from build123d import *

# Parameters (mm, degrees)
BOSS_EXTRUDE1_DEPTH = 6
SKETCH2_R           = 7.5
BOSS_EXTRUDE2_DEPTH = 24
BOSS_EXTRUDE3_DEPTH = 6
SKETCH4_R           = 6.75
CUT_EXTRUDE1_DEPTH  = 44.338781709
SKETCH5_R           = 2.25
CUT_EXTRUDE2_DEPTH  = 13
CHAMFER1_SIZE       = 1
CHAMFER2_SIZE       = 2
SKETCH6_R           = 2
CUT_EXTRUDE3_DEPTH  = 44.338781709


with BuildPart() as part:
    # Sketch1 → Boss-Extrude1 (new body)
    with BuildSketch(Plane.XY):
        with BuildLine():
            Line((-13.5, 0), (-13.5, -20))
            Line((-13.5, -20), (13.5, -20))
            Line((13.5, -20), (13.5, 0))
            ThreePointArc((13.5, 0), (0, 13.5), (-13.5, 0))
        make_face()
    extrude(amount=BOSS_EXTRUDE1_DEPTH)

    # Sketch2 → Boss-Extrude2 (add)
    with BuildSketch(Plane.XY.offset(6)):
        Circle(SKETCH2_R)
    extrude(amount=BOSS_EXTRUDE2_DEPTH)

    # Sketch3 → Boss-Extrude3 (add)
    with BuildSketch(Plane.XY.offset(30)):
        with BuildLine():
            Line((-13.5, 0), (-13.5, -20))
            Line((-13.5, -20), (13.5, -20))
            Line((13.5, -20), (13.5, 0))
            ThreePointArc((13.5, 0), (0, 13.5), (-13.5, 0))
        make_face()
    extrude(amount=BOSS_EXTRUDE3_DEPTH)

    # Sketch4 → Cut-Extrude1 (cut, through all)
    with BuildSketch(Plane.XY.offset(36)):
        Circle(SKETCH4_R)
    extrude(amount=-CUT_EXTRUDE1_DEPTH, mode=Mode.SUBTRACT)

    # Sketch5 → Cut-Extrude2 (cut)
    with BuildSketch(Plane.XZ.offset(20)):
        with Locations((-5, 33)):
            Circle(SKETCH5_R)
        with Locations((5, 33)):
            Circle(SKETCH5_R)
        with Locations((-5, 3)):
            Circle(SKETCH5_R)
        with Locations((5, 3)):
            Circle(SKETCH5_R)
    extrude(amount=-CUT_EXTRUDE2_DEPTH, mode=Mode.SUBTRACT)

    # Chamfer1
    # the kernel refuses this chamfer: 1 mm, written as the material it takes off along each edge
    with BuildSketch(Plane(origin=(5, -20, 33), x_dir=(1, 0, 0), z_dir=(0, 0, -1))) as chamfer1_piece_1:
        Polygon((2.25 + CHAMFER1_SIZE, 0), (2.25, -CHAMFER1_SIZE), (2.25, 0), align=None)
    revolve(axis=Axis((5, -20, 33), (0, -1, 0)), mode=Mode.SUBTRACT)
    with BuildSketch(Plane(origin=(-5, -20, 3), x_dir=(1, 0, 0), z_dir=(0, 0, -1))) as chamfer1_piece_2:
        Polygon((2.25 + CHAMFER1_SIZE, 0), (2.25, -CHAMFER1_SIZE), (2.25, 0), align=None)
    revolve(axis=Axis((-5, -20, 3), (0, -1, 0)), mode=Mode.SUBTRACT)
    with BuildSketch(Plane(origin=(5, -20, 3), x_dir=(1, 0, 0), z_dir=(0, 0, -1))) as chamfer1_piece_3:
        Polygon((2.25 + CHAMFER1_SIZE, 0), (2.25, -CHAMFER1_SIZE), (2.25, 0), align=None)
    revolve(axis=Axis((5, -20, 3), (0, -1, 0)), mode=Mode.SUBTRACT)
    with BuildSketch(Plane(origin=(-5, -20, 33), x_dir=(1, 0, 0), z_dir=(0, 0, -1))) as chamfer1_piece_4:
        Polygon((2.25 + CHAMFER1_SIZE, 0), (2.25, -CHAMFER1_SIZE), (2.25, 0), align=None)
    revolve(axis=Axis((-5, -20, 33), (0, -1, 0)), mode=Mode.SUBTRACT)

    # Chamfer2
    chamfer2_edges = [part.edges().sort_by_distance(p)[0] for p in [
        (13.5, -10, 6),
        (0, 13.5, 30),
        (-13.5, -10, 30),
        (13.5, -10, 30),
        (0, 13.5, 36),
        (-13.5, -10, 36),
        (13.5, -10, 36),
        (0, 13.5, 6),
        (13.5, -10, 0),
        (-13.5, -10, 0),
        (0, 13.5, 0),
        (-13.5, -10, 6),
    ]]
    chamfer(chamfer2_edges, length=CHAMFER2_SIZE)

    # Sketch6 → Cut-Extrude3 (cut, through all)
    with BuildSketch(Plane.XY.offset(36)):
        with Locations(Location((-10, 0, 0), (0, 0, 221.409622109))):
            Circle(SKETCH6_R)
    extrude(amount=-CUT_EXTRUDE3_DEPTH, mode=Mode.SUBTRACT)


solid = part.part
The model under review builds one solid part; all positions refer to its coordinate system, in mm. A direction names the side the tool comes from. Round coordinates to 2 decimals unless told otherwise and drop trailing zeros. Write each loop counter-clockwise with the first axis right and the second up, starting at its lowest first coordinate (ties: lowest second). Pieces come first, ordered by that corner, then holes. Notation, with made-up numbers: M 59.25,38 L 101.25,38 A23 cw 101.25,59 Z; hole C 9,37 d7. An arc over 180 degrees is marked long. Use a Markdown table: item, result. Add a question column.
Q1. Insertion check: pin 1 (2.5 mm diameter, centred on x = -5, z = 33, fed in from -Y); pin 2 (7 mm diameter, centred on x = 5, z = 3, fed in from -Y); pin 3 (2 mm diameter, centred on x = -4, z = 4, fed in from -Y); pin 4 (10 mm diameter, centred on y = -4, z = 11.5, fed in from +X). Each pin has a flat end and moves straight along its axis. Give the tip position at first contact, or say it passes through.
Q2. To check wall thickness, follow line 1 (Z direction, x = -5, y = -10.75); line 2 (X direction, y = -18.5, z = 2.5); line 3 (Y direction, x = 0, z = 15.5). State the ranges of each line that lie inside material, in increasing order.
Q3. We need section B-B, the plane z = 33. State the section outline as (x, y) points.
Q4. We need section A-A, the plane y = -16.5. State the section outline as (x, z) points, plus the area to 3 significant figures.
Q5. We need section C-C, the plane y = -3. State the section outline as (x, z) points, plus the area to 3 significant figures.
Q6. The part is to be moulded in two halves that separate along Z. For faces 4 (the face through (0, -8, 0)), 5 (the face through (-13.5, -10, 3)), 6 (the face through (5, -7, 3)), say which applies: pulls with the +Z half, pulls with the -Z half, needs draft (parallel to the pull), parting line crosses it, or undercut.
Q7. Machinability: for faces 1 (the face through (0, -8, 30)), 2 (the face through (0.26, 11.816, 30.319)), 3 (the face through (5, -7, 33)), which of the approach directions +Z, -Z, +X, -X, +Y, -Y give a long, thin tool a straight path to every point of the face, cutting with its end or side? Answer none if there is none.
Q8. We need section D-D, the plane z = 27.5. State the section outline as (x, y) points, plus the area to 3 significant figures.
Findings below:
| question | item | result |
|---|---|---|
| 1 | pin 1 | stops at y = -7 |
| 1 | pin 2 | stops at y = -20 |
| 1 | pin 3 | stops at y = -19.16 |
| 1 | pin 4 | stops at x = 7.5 |
| 2 | line 1 | z = 0 to 0.75, 5.25 to 6, 30 to 30.75, 35.25 to 36 |
| 2 | line 2 | x = -13.5 to -7.19, -2.81 to 2.81, 7.19 to 13.5 |
| 2 | line 3 | y = -7.5 to -6.75, 6.75 to 7.5 |
| 3 | outline | M -13.5,-20 L -8.25,-20 L -7.25,-19 L -7.25,-7 L -2.75,-7 L -2.75,-19 L -1.75,-20 L 1.75,-20 L 2.75,-19 L 2.75,-7 L 7.25,-7 L 7.25,-19 L 8.25,-20 L 13.5,-20 L 13.5,0 A13.5 ccw -13.5,0 Z; hole C -10,0 d4; hole C 0,0 d13.5 |
| 4 | outline | M -13.5,2 L -11.5,0 L 11.5,0 L 13.5,2 L 13.5,4 L 11.5,6 L -11.5,6 L -13.5,4 Z; M -13.5,32 L -11.5,30 L 11.5,30 L 13.5,32 L 13.5,34 L 11.5,36 L -11.5,36 L -13.5,34 Z; hole C -5,3 d4.5; hole C -5,33 d4.5; hole C 5,3 d4.5; hole C 5,33 d4.5 |
| 4 | area | 244 mm² |
| 5 | outline | M -13.5,2 L -11.5,0 L -6.05,0 L -6.05,36 L -11.5,36 L -13.5,34 L -13.5,32 L -11.5,30 L -6.87,30 L -6.87,6 L -11.5,6 L -13.5,4 Z; M 6.05,0 L 11.5,0 L 13.5,2 L 13.5,4 L 11.5,6 L 6.87,6 L 6.87,30 L 11.5,30 L 13.5,32 L 13.5,34 L 11.5,36 L 6.05,36 Z |
| 5 | area | 203 mm² |
| 6 | face 4 | pulls with the -Z half |
| 6 | face 5 | needs draft |
| 6 | face 6 | undercut |
| 7 | face 1 | none |
| 7 | face 2 | +Y |
| 7 | face 3 | -Y |
| 8 | outline | C 0,0 d15; hole C 0,0 d13.5 |
| 8 | area | 33.6 mm² |
